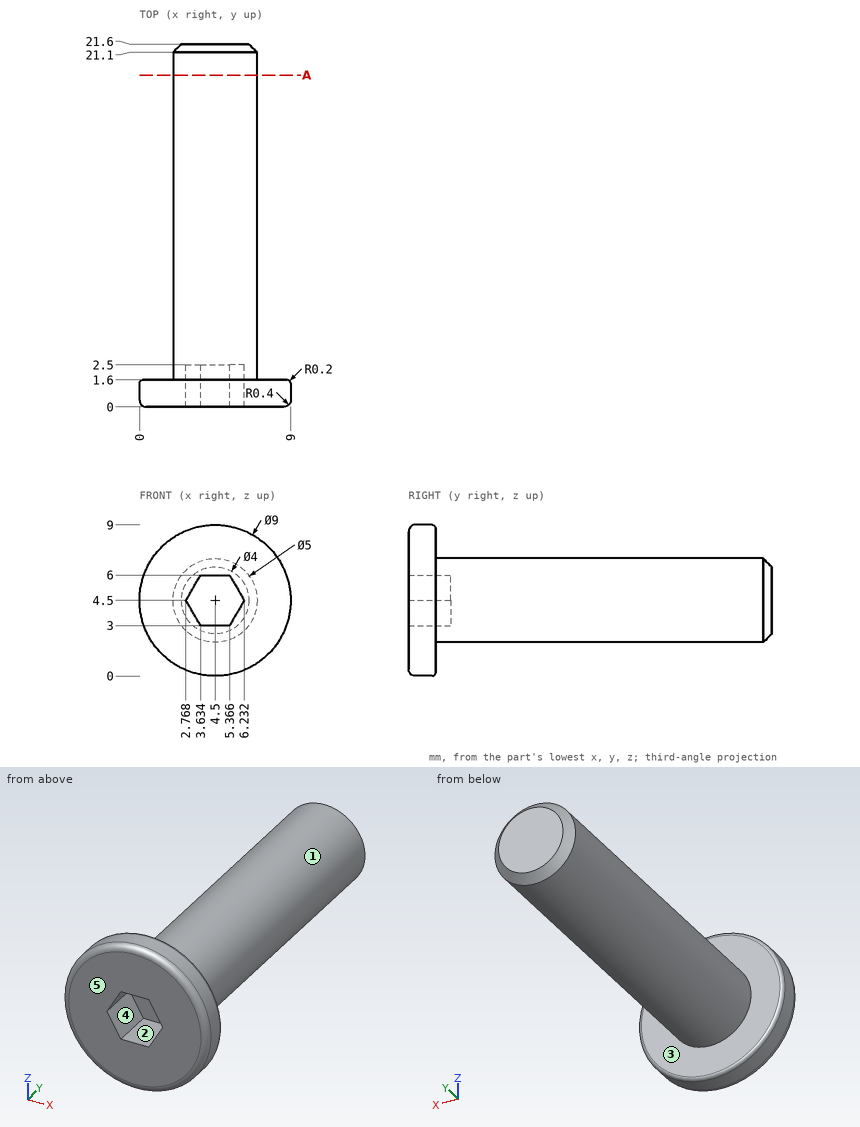
For this review, use the dimensioned drawing (mm, ordinates from the lowest corner) and the shaded views. A direction names the side the tool comes from. Round coordinates to 2 decimals unless told otherwise and drop trailing zeros. Write each loop counter-clockwise with the first axis right and the second up, starting at its lowest first coordinate (ties: lowest second). Pieces come first, ordered by that corner, then holes. Notation, with made-up numbers: (76.25, -17.5) -> (124.25, -17.5) arc R5 ccw to (124.25, -9.5) -> close; hole circle Ø6 at (-20.5, 30). An arc over 180 degrees is marked (long way). One line per item, written item: value. Start each with the question number.
Q1. Add section A-A (y = 19.75). Give the boundary of the cut face in (x, z).
Q2. Insertion check: P1, Ø5, axis at y = 9, z = 1.5, coming from the +X side; P2, Ø5, axis at x = 6, y = 16, coming from the -Z side; P3, Ø1.5, axis at x = 5, z = 4.5, coming from the -Y side; P4, Ø1.5, axis at x = 8, y = 18.5, coming from the +Z side. Each pin has a flat end and moves straight along its axis. Give the tip position at first contact, or say it passes through.
Q3. To check wall thickness, follow probe 1 along Z at (x, y) = (4.5, 18.25); probe 2 along Y at (x, z) = (4.25, 8.5); probe 3 along Y at (x, z) = (6, 4.75). State the ranges of each line that lie inside material, in increasing order.
Q4. Tool access review of the marked faces 4 and 5: name each direction out of +Z, -Z, +X, -X, +Y, -Y from which nothing blocks a thin tool from reaching the whole face with its end or side.
Q5. The part is to be moulded in two halves that separate along X. For the marked faces 1, 2 and 3, say which applies: pulls with the +X half, pulls with the -X half, needs draft (parallel to the pull), parting line crosses it, or undercut.
Response:
1. outline: circle Ø5 at (4.5, 4.5)
2. P1: stops at x = 6.95
2. P2: stops at z = 2
2. P3: stops at y = 2.5
2. P4: passes through
3. probe 1: z = 2 to 7
3. probe 2: y = 0 to 1.6
3. probe 3: y = 2.5 to 21.6
4. face 4: -Y
4. face 5: +Z, -Z, +X, -X, -Y
5. face 1: parting line crosses it
5. face 2: undercut
5. face 3: needs draft
